```python
from build123d import *


with BuildPart() as f1:
    # F0 (on Front) → F1 (revolve)
    with BuildSketch(Plane.XZ):
        with BuildLine():
            Line((55, 0), (0, 0))
            Line((0, 0), (0, -10))
            Line((0, -10), (3.5, -10))
            Line((3.5, -10), (6.5, -9))
            Line((6.5, -9), (9.5, -10))
            Line((9.5, -10), (13, -10))
            ThreePointArc((13, -10), (15.12132, -9.12132), (16, -7))
            Line((16, -7), (22, -7))
            ThreePointArc((22, -7), (22.585786, -5.585786), (24, -5))
            Line((24, -5), (38, -5))
            ThreePointArc((38, -5), (39.414214, -5.585786), (40, -7))
            Line((40, -7), (43, -7))
            ThreePointArc((43, -7), (43.292893, -7.707107), (44, -8))
            Line((44, -8), (52, -8))
            ThreePointArc((52, -8), (54.12132, -7.12132), (55, -5))
            Line((55, -5), (55, 0))
        make_face()
    revolve(axis=Axis((24.909981, 0, 0), (-1, 0, 0)))


solid = f1.part
```
Here's how the part is built. I have some questions about the finished solid (model axes, mm). A direction names the side the tool comes from. Coordinates: 2 decimals unless noted, no trailing zeros. Order: outer loops, then holes, each group sorted by start corner. A loop starts at its lowest first (then second) coordinate and runs counter-clockwise, first axis right, second up.
Item 1: If we section it at C-C, the plane x = 33.5: List the corners of the cut face in (y, z) for me, then the cut area to 3 significant figures.
Response values:
outline: circle Ø10 at (0, 0)
area: 78.5 mm2
Item 2: Which directions (+Z, -Z, +X, -X, +Y, -Y) give clear straight access to the entire face, cutting with the end or side of a thin tool? Please do faces 1 (the face through (1.77, 9.76, 2.17)), 2 (the face through (6.354, 8.833, 1.962)), 3 (the face through (48.06, 7.81, 1.73)).
Response values:
face 1: +X, -X
face 2: none
face 3: +X
Item 3: Thinking about a two-plate mould opening in X: for faces 4 (the face through (0, 0, 0)), 5 (the face through (41.521, 2.681, -6.466)), 6 (the face through (11.27, 9.76, 2.17)), which applies, pulls with the +X half, pulls with the -X half, needs draft (parallel to the pull), parting line crosses it, or undercut?
Response values:
face 4: pulls with the -X half
face 5: undercut
face 6: needs draft
Item 4: I need wall thicknesses on probe 1 along X at (y, z) = (0.25, 7.25); probe 2 along X at (y, z) = (-3.75, -5.5); probe 3 along Z at (x, y) = (7.5, -6.25). Which ranges of each line are inside material? Lowest first, please.
Response values:
probe 1: x = 0 to 15.99, 43.03 to 53.98
probe 2: x = 0 to 22.03, 39.97 to 54.5
probe 3: z = -6.93 to 6.93
Item 5: I'm going to push flat-ended pins straight in: pin 1 Ø1.5 at (x, y) = (10.5, -6) entering from +Z; pin 2 Ø3 at (x, z) = (32, 2.5) entering from -Y; pin 3 Ø4 at (x, y) = (15.5, -3) entering from -Z. Where does each tip first touch, or does it pass through?
Response values:
pin 1: stops at z = 8.51
pin 2: stops at y = -4.9
pin 3: stops at z = -9.7
Item 6: If we section it at A-A, the plane z = 0: List the corners of the cut face in (x, y) for me, then the cut area to 3 significant figures.
Response values:
outline: (0, -10) - (3.5, -10) - (6.5, -9) - (9.5, -10) - (13, -10) arc R3 ccw to (16, -7) - (22, -7) arc R2 cw to (24, -5) - (38, -5) arc R2 cw to (40, -7) - (43, -7) arc R1 ccw to (44, -8) - (52, -8) arc R3 ccw to (55, -5) - (55, 5) arc R3 ccw to (52, 8) - (44, 8) arc R1 ccw to (43, 7) - (40, 7) arc R2 cw to (38, 5) - (24, 5) arc R2 cw to (22, 7) - (16, 7) arc R3 ccw to (13, 10) - (9.5, 10) - (6.5, 9) - (3.5, 10) - (0, 10) - close
area: 807 mm2
Item 7: If we section it at D-D, the plane x = 23.5: List the corners of the cut face in (y, z) for me, then the cut area to 3 significant figures.
Response values:
outline: circle Ø10.13 at (0, 0)
area: 80.5 mm2
